from build123d import *

# Parameters (mm, degrees)
F1_DEPTH = 6.35
F3_DEPTH = 30.48


with BuildPart() as f1:
    # F0 (on Top) → F1 (new body)
    with BuildSketch(Plane.XY):
        with BuildLine():
            Line((-4.9193716261, 40.5964435692), (-8.8563716261, 40.5964435692))
            Line((-8.8563716261, 40.5964435692), (-8.8563716261, 38.2469435692))
            ThreePointArc((-8.8563716261, 38.2469435692), (-5.5606176297, 36.8817975657), (-4.1954716261, 33.5860435692))
            Line((-4.1954716261, 33.5860435692), (-0.8299716261, 33.5860435692))
            Line((-0.8299716261, 33.5860435692), (-4.9193716261, 40.5964435692))
        make_face()
        with BuildLine():
            Line((-8.8563716261, 38.2469435692), (-8.8563716261, 40.5964435692))
            Line((-8.8563716261, 40.5964435692), (-12.7933716261, 40.5964435692))
            Line((-12.7933716261, 40.5964435692), (-16.8827716261, 33.5860435692))
            Line((-16.8827716261, 33.5860435692), (-13.5172716261, 33.5860435692))
            ThreePointArc((-13.5172716261, 33.5860435692), (-12.1521256225, 36.8817975657), (-8.8563716261, 38.2469435692))
        make_face()
        with BuildLine():
            ThreePointArc((-8.8563716261, 28.9251435692), (-12.1521256225, 30.2902895728), (-13.5172716261, 33.5860435692))
            Line((-13.5172716261, 33.5860435692), (-16.8827716261, 33.5860435692))
            Line((-16.8827716261, 33.5860435692), (-12.7933716261, 26.5756435692))
            Line((-12.7933716261, 26.5756435692), (-8.8563716261, 26.5756435692))
            Line((-8.8563716261, 26.5756435692), (-8.8563716261, 28.9251435692))
        make_face()
        with BuildLine():
            Line((-0.8299716261, 33.5860435692), (-4.1954716261, 33.5860435692))
            ThreePointArc((-4.1954716261, 33.5860435692), (-5.5606176297, 30.2902895728), (-8.8563716261, 28.9251435692))
            Line((-8.8563716261, 28.9251435692), (-8.8563716261, 26.5756435692))
            Line((-8.8563716261, 26.5756435692), (-4.9193716261, 26.5756435692))
            Line((-4.9193716261, 26.5756435692), (-0.8299716261, 33.5860435692))
        make_face()
        with BuildLine():
            Line((-8.8563716261, 33.5860435692), (-8.8563716261, 38.2469435692))
            ThreePointArc((-8.8563716261, 38.2469435692), (-12.1521256225, 36.8817975657), (-13.5172716261, 33.5860435692))
            Line((-13.5172716261, 33.5860435692), (-8.8563716261, 33.5860435692))
        make_face()
        with BuildLine():
            ThreePointArc((-4.1954716261, 33.5860435692), (-5.5606176297, 36.8817975657), (-8.8563716261, 38.2469435692))
            Line((-8.8563716261, 38.2469435692), (-8.8563716261, 33.5860435692))
            Line((-8.8563716261, 33.5860435692), (-4.1954716261, 33.5860435692))
        make_face()
        with BuildLine():
            Line((-4.1954716261, 33.5860435692), (-8.8563716261, 33.5860435692))
            Line((-8.8563716261, 33.5860435692), (-8.8563716261, 28.9251435692))
            ThreePointArc((-8.8563716261, 28.9251435692), (-5.5606176297, 30.2902895728), (-4.1954716261, 33.5860435692))
        make_face()
        with BuildLine():
            Line((-8.8563716261, 28.9251435692), (-8.8563716261, 33.5860435692))
            Line((-8.8563716261, 33.5860435692), (-13.5172716261, 33.5860435692))
            ThreePointArc((-13.5172716261, 33.5860435692), (-12.1521256225, 30.2902895728), (-8.8563716261, 28.9251435692))
        make_face()
    extrude(amount=-F1_DEPTH)

    # F2 (on face) → F3 (join)
    with BuildSketch(Plane.XY):
        with BuildLine():
            Line((-13.5045716261, 33.5860435692), (-4.2081716261, 33.5860435692))
            ThreePointArc((-4.2081716261, 33.5860435692), (-8.8563716261, 38.2342435692), (-13.5045716261, 33.5860435692))
        make_face()
        with BuildLine():
            ThreePointArc((-13.5045716261, 33.5860435692), (-8.8563716261, 28.9378435692), (-4.2081716261, 33.5860435692))
            Line((-4.2081716261, 33.5860435692), (-13.5045716261, 33.5860435692))
        make_face()
    extrude(amount=F3_DEPTH)


solid = f1.part
Could you check a few things on this model? Use its own coordinates, in mm. A direction names the side the tool comes from. Coordinates: 2 decimals unless noted, no trailing zeros. Loops run counter-clockwise (first coordinate to the right, second up) from the corner with the lowest first, then second, coordinate; pieces in that order, holes last.
1. Imagine slicing it at A-A (x = -6.75). Please give me the cut outline in (y, z).
2. For P1, Ø6, axis at x = -3, y = 34, coming from the +Z side; P2, Ø3, axis at y = 30, z = 17.5, coming from the -X side; P3, Ø4, axis at x = -5, z = 19, coming from the -Y side; P4, Ø1, axis at x = -12, z = 4.5, coming from the -Y side, each with a flat end and sliding along its axis, tell me the tip position at first contact or that it passes through.
3. For faces 1 (the face through (-2.846, 37.042, -3.131)), 2 (the face through (-8.251, 28.977, 15.027)), which set-ups out of +Z, -Z, +X, -X, +Y, -Y let a thin tool reach every point of the face, with its end or its side?
4. Imagine slicing it at C-C (y = 37.25). Please give me the cut outline in (x, z).
5. Imagine slicing it at D-D (z = 21). Please give me the cut outline in (x, y).
6. I need wall thicknesses on L1, parallel to Z at x = -14.5, y = 31; L2, parallel to X at y = 33.5, z = 20; L3, parallel to X at y = 39.75, z = -0.5. Which ranges of each line are inside material? Lowest first, please.
7. Imagine slicing it at B-B (z = -1). Please give me the cut outline in (x, y), and give its area (3 significant figures).
Computed values:
1. outline: (26.58, -6.35) - (40.6, -6.35) - (40.6, 0) - (37.73, 0) - (37.73, 30.48) - (29.44, 30.48) - (29.44, 0) - (26.58, 0) - close
2. P1: stops at z = 30.48
2. P2: stops at x = -13.01
2. P3: stops at y = 29.32
2. P4: stops at y = 29.76
3. face 1: +Z, -Z, +X, +Y
3. face 2: +Z
4. outline: (-14.75, -6.35) - (-2.97, -6.35) - (-2.97, 0) - (-6, 0) - (-6, 30.48) - (-11.72, 30.48) - (-11.72, 0) - (-14.75, 0) - close
5. outline: circle Ø9.3 at (-8.86, 33.59)
6. L1: z = -6.35 to 0
6. L2: x = -13.5 to -4.21
6. L3: x = -13.29 to -4.43
7. outline: (-16.88, 33.59) - (-12.79, 26.58) - (-4.92, 26.58) - (-0.83, 33.59) - (-4.92, 40.6) - (-12.79, 40.6) - close
7. area: 168 mm2
